```python
from build123d import *

# Parameters (mm, degrees)
F0_W     = 5.5
F0_H     = 7
F0_R     = 2
F1_DEPTH = 2
F2_R     = 5


with BuildPart() as f1:
    # F0 (on Top) → F1 (new body)
    with BuildSketch(Plane.XY):
        Polygon((21, 8.5), (10.5, 8.5), (-10.5, 8.5), (-21, 8.5), (-21, -8.5), (-10.5, -8.5), (10.5, -8.5), (21, -8.5), align=None)
        Polygon((16, -3.5), (10.5, -3.5), (-10.5, -3.5), (-16, -3.5), (-16, 3.5), (-10.5, 3.5), (10.5, 3.5), (16, 3.5), align=None, mode=Mode.SUBTRACT)
        with Locations((-13.25, 0)):
            Rectangle(F0_W, F0_H)
        with Locations((-13.6, 0)):
            Circle(F0_R, mode=Mode.SUBTRACT)
        with Locations((13.25, 0)):
            Rectangle(F0_W, F0_H)
        with Locations((13.6, 0)):
            Circle(F0_R, mode=Mode.SUBTRACT)
    extrude(amount=F1_DEPTH)

    # F2
    f2_edges = [f1.edges().sort_by_distance(p)[0] for p in [
        (-21, 8.5, 1),
        (-21, -8.5, 1),
        (21, -8.5, 1),
        (21, 8.5, 1),
    ]]
    fillet(f2_edges, radius=F2_R)


solid = f1.part
```
Part model, mm, in its own coordinate system. A direction names the side the tool comes from. Give positions to 0.01 mm unless a question says otherwise; leave off trailing zeros. Write each loop counter-clockwise with the first axis right and the second up, starting at its lowest first coordinate (ties: lowest second). Pieces come first, ordered by that corner, then holes. Notation, with made-up numbers: (64, 80.5) -> (83, 80.5) arc R11 cw to (83, 101.5) -> close; hole circle Ø1 at (47, 2). An arc over 180 degrees is marked (long way). Put each result on its own line as item: value. Start each with the question number.
Item 1: Pull direction X, two halves, no side cores. Call faces 3 (the face through (0, -4, 0)), 4 (the face through (-10.5, 0, 1)), 5 (the face through (21, 0, 1)), 6 (the face through (-19.57, -7, 1.01)): pulls with the +X half, pulls with the -X half, needs draft (parallel to the pull), parting line crosses it, or undercut.
Item 2: Wall check: L1, parallel to Y at x = -0.5, z = 0.5; L2, parallel to Y at x = 13.6, z = 0.5; L3, parallel to X at y = -3.25, z = 1.8. Give the ranges that are in metal, low to high. Write a range as [from, to].
Item 3: Cut at A-A (y = 0). List the corners of the cut face in (x, z).
Item 4: Which spindle directions (+Z, -Z, +X, -X, +Y, -Y) get a long thin tool onto all of the face, cutting with end or side? Do faces 1 (the face through (0, -3.5, 1)), 2 (the face through (19.5, 7.07, 1.01)). Say none if no direction does.
Item 5: Cut at B-B (x = 7). List the corners of the cut face in (y, z).
Item 6: Cut at D-D (x = -13.6). List the corners of the cut face in (y, z), then the cut area to 3 significant figures.
Item 7: Cut at C-C (z = 0.35). List the corners of the cut face in (x, y).
Answer list:
1. face 3: needs draft
1. face 4: undercut
1. face 5: pulls with the +X half
1. face 6: pulls with the -X half
2. L1: y = [-8.5, -3.5], [3.5, 8.5]
2. L2: y = [-8.5, -2], [2, 8.5]
2. L3: x = [-21, -10.5], [10.5, 21]
3. outline: (-21, 0) -> (-15.6, 0) -> (-15.6, 2) -> (-21, 2) -> close; (-11.6, 0) -> (-10.5, 0) -> (-10.5, 2) -> (-11.6, 2) -> close; (10.5, 0) -> (11.6, 0) -> (11.6, 2) -> (10.5, 2) -> close; (15.6, 0) -> (21, 0) -> (21, 2) -> (15.6, 2) -> close
4. face 1: +Z, -Z
4. face 2: +Z, -Z, +X, +Y
5. outline: (-8.5, 0) -> (-3.5, 0) -> (-3.5, 2) -> (-8.5, 2) -> close; (3.5, 0) -> (8.5, 0) -> (8.5, 2) -> (3.5, 2) -> close
6. outline: (-8.5, 0) -> (-2, 0) -> (-2, 2) -> (-8.5, 2) -> close; (2, 0) -> (8.5, 0) -> (8.5, 2) -> (2, 2) -> close
6. area: 26.0 mm2
7. outline: (-21, -3.5) arc R5 ccw to (-16, -8.5) -> (16, -8.5) arc R5 ccw to (21, -3.5) -> (21, 3.5) arc R5 ccw to (16, 8.5) -> (-16, 8.5) arc R5 ccw to (-21, 3.5) -> close; hole circle Ø4 at (-13.6, 0); hole (-10.5, -3.5) -> (10.5, -3.5) -> (10.5, 3.5) -> (-10.5, 3.5) -> close; hole circle Ø4 at (13.6, 0)
